Source: CAD feature listing. Evaluate the final solid. Frame: model axes, mm. A direction names the side the tool comes from. Round coordinates to 2 decimals unless told otherwise and drop trailing zeros. Loops run counter-clockwise (first coordinate to the right, second up) from the corner with the lowest first, then second, coordinate; pieces in that order, holes last. Notation, with made-up numbers: (-27.75, -29) -> (-13.75, -29) arc R32 ccw to (-13.75, 4) -> close; hole circle Ø9 at (10, -13). An arc over 180 degrees is marked (long way). Put each result on its own line as item: value. Start each with the question number.
1. Cut plane D-D (y = 9.5). Return the cut outline in (x, z), then the cut area to 3 significant figures.
2. Draft query along Y for faces 1 (the flat face through (0, -15, 1)), 2 (the cylindrical face through (13.2, -10.5, 1)), 3 (the flat face through (-10, 0, 10)). Return one class per face: pulls with the +Y half, pulls with the -Y half, needs draft (parallel to the pull), parting line crosses it, or undercut.
3. Cut plane A-A (y = 13). Return the cut outline in (x, z), then the cut area to 3 significant figures.
4. Contact query for flat-ended pins moving along their axis: pin 1 (2 mm diameter, centred on x = -13, z = 1.5, fed in from -Y); pin 2 (2.5 mm diameter, centred on y = 8, z = 8, fed in from -X); pin 3 (3 mm diameter, centred on x = -14, y = 13, fed in from -Z); pin 4 (1.5 mm diameter, centred on y = -5.5, z = 8, fed in from +X). Output: stop coordinate, or through.
5. Cut plane C-C (z = 9.25). Return the cut outline in (x, y).
6. Cut plane B-B (x = -14). Return the cut outline in (y, z).
7. Material intervals for L1, parallel to Y at x = -14, z = 0.65; L2, parallel to X at y = 11, z = 3.5; L3, parallel to Z at x = -5.5, y = -9, sorted ascending.
8. Set-up query: faces 4 (the flat face through (0, -14, 3)), 5 (the flat face through (13, -12, 1)), 6 (the flat face through (0, -15, 4)), 7 (the flat face through (-14, 2, 2)), 8 (the flat face through (-13, -12, 1)). Return all of +Z, -Z, +X, -X, +Y, -Y with unobstructed straight access to the full face (end or side cutting, diameter ignored); none if empty.
```python
from build123d import *

# Parameters (mm, degrees)
SKETCH1_W                = 34
SKETCH1_H                = 32
BOSS_EXTRUDE1_DEPTH      = 2
SKETCH2_W                = 2.6
SKETCH2_H                = 2
BOSS_EXTRUDE2_DEPTH      = 8
SKETCH2_4_W              = 12.8
SKETCH2_4_H              = 2
BOSS_EXTRUDE3_DEPTH      = 2
SKETCH3_W                = 6
SKETCH3_H                = 4
CUT_EXTRUDE1_DEPTH       = 9
M3_CLEARANCE_HOLE1_D     = 3.4
M3_CLEARANCE_HOLE1_DEPTH = 10
M3_CLEARANCE_HOLE1_TIP   = 1.021463052
FILLET1_R                = 1.5
CHAMFER1_SIZE            = 2
FILLET2_R                = 1.5


with BuildPart() as part:
    # Sketch1 → Boss-Extrude1 (new body)
    with BuildSketch(Plane.XY):
        Rectangle(SKETCH1_W, SKETCH1_H)
    extrude(amount=BOSS_EXTRUDE1_DEPTH)

    # Sketch2 → Boss-Extrude2 (add)
    with BuildSketch(Plane.XY.offset(2)):
        Polygon((11, 16), (9, 16), (9, -14), (9, -16), (11, -16), align=None)
        Polygon((-9, 16), (-11, 16), (-11, -16), (-9, -16), (-9, -14), align=None)
        with Locations((-7.7, -15)):
            Rectangle(SKETCH2_W, SKETCH2_H)
        with Locations((7.7, -15)):
            Rectangle(SKETCH2_W, SKETCH2_H)
    extrude(amount=BOSS_EXTRUDE2_DEPTH)

    # Sketch2_4 → Boss-Extrude3 (add)
    with BuildSketch(Plane.XY.offset(2)):
        with Locations((0, -15)):
            Rectangle(SKETCH2_4_W, SKETCH2_4_H)
    extrude(amount=BOSS_EXTRUDE3_DEPTH)

    # Sketch3 → Cut-Extrude1 (cut)
    with BuildSketch(Plane.XY.offset(2)):
        with Locations((-14, -14)):
            Rectangle(SKETCH3_W, SKETCH3_H)
        with Locations((14, -14)):
            Rectangle(SKETCH3_W, SKETCH3_H)
    extrude(amount=-CUT_EXTRUDE1_DEPTH, mode=Mode.SUBTRACT)

    # M3 Clearance Hole1
    with Locations(Plane.XY.offset(2)):
        with Locations((-14, 13), (14, -9), (-14, -9), (14, 13)):
            Hole(M3_CLEARANCE_HOLE1_D / 2, depth=M3_CLEARANCE_HOLE1_DEPTH)
            with Locations((0, 0, -(M3_CLEARANCE_HOLE1_DEPTH + M3_CLEARANCE_HOLE1_TIP / 2))):  # 118° drill point
                Cone(0, M3_CLEARANCE_HOLE1_D / 2, M3_CLEARANCE_HOLE1_TIP, mode=Mode.SUBTRACT)

    # Fillet1
    fillet1_edges = [part.edges().sort_by_distance(p)[0] for p in [
        (-17, 16, 1),
        (17, 16, 1),
        (-17, -12, 1),
        (17, -12, 1),
    ]]
    fillet(fillet1_edges, radius=FILLET1_R)

    # Chamfer1
    chamfer1_edges = [part.edges().sort_by_distance(p)[0] for p in [
        (0, -16, 0),
    ]]
    chamfer(chamfer1_edges, length=CHAMFER1_SIZE)

    # Fillet2
    fillet2_edges = [part.edges().sort_by_distance(p)[0] for p in [
        (0, -16, 2),
    ]]
    fillet(fillet2_edges, radius=FILLET2_R)


solid = part.part
```
Solution:
1. outline: (-17, 0) -> (17, 0) -> (17, 2) -> (11, 2) -> (11, 10) -> (9, 10) -> (9, 2) -> (-9, 2) -> (-9, 10) -> (-11, 10) -> (-11, 2) -> (-17, 2) -> close
1. area: 100 mm^2
2. face 1: pulls with the -Y half
2. face 2: undercut
2. face 3: needs draft
3. outline: (-17, 0) -> (-15.7, 0) -> (-15.7, 2) -> (-17, 2) -> close; (-12.3, 0) -> (12.3, 0) -> (12.3, 2) -> (11, 2) -> (11, 10) -> (9, 10) -> (9, 2) -> (-9, 2) -> (-9, 10) -> (-11, 10) -> (-11, 2) -> (-12.3, 2) -> close; (15.7, 0) -> (17, 0) -> (17, 2) -> (15.7, 2) -> close
3. area: 86.4 mm^2
4. pin 1: stops at y = -12
4. pin 2: stops at x = -11
4. pin 3: passes through
4. pin 4: stops at x = 11
5. outline: (-11, -16) -> (-6.4, -16) -> (-6.4, -14) -> (-9, -14) -> (-9, 16) -> (-11, 16) -> close; (6.4, -16) -> (11, -16) -> (11, 16) -> (9, 16) -> (9, -14) -> (6.4, -14) -> close
6. outline: (-12, 0) -> (-10.7, 0) -> (-10.7, 2) -> (-12, 2) -> close; (-7.3, 0) -> (11.3, 0) -> (11.3, 2) -> (-7.3, 2) -> close; (14.7, 0) -> (16, 0) -> (16, 2) -> (14.7, 2) -> close
7. L1: y = -12 to -10.7, -7.3 to 11.3, 14.7 to 16
7. L2: x = -11 to -9, 9 to 11
7. L3: z = 0 to 2
8. face 4: +Z, +Y
8. face 5: +Z, -Z, +X, -Y
8. face 6: +Z, +Y, -Y
8. face 7: +Z, -X, +Y, -Y
8. face 8: +Z, -Z, -X, -Y
